```python
from build123d import *

# Parameters (mm, degrees)
CROQUIS1_W              = 43
CROQUIS1_H              = 15.5
SALIENTE_EXTRUIR1_DEPTH = 2
SALIENTE_EXTRUIR2_START = -2
SALIENTE_EXTRUIR2_DEPTH = 2


with BuildPart() as part:
    # Croquis1 → Saliente-Extruir1 (new body)
    with BuildSketch(Plane(origin=(0, 0, 0), x_dir=(1, 0, 0), z_dir=(0, 1, 0))):
        with BuildLine():
            Line((-24.5, 8.75), (-24.5, -8.75))
            ThreePointArc((-24.5, -8.75), (-23.914213562, -10.164213562), (-22.5, -10.75))
            Line((-22.5, -10.75), (22.5, -10.75))
            ThreePointArc((22.5, -10.75), (23.914213562, -10.164213562), (24.5, -8.75))
            Line((24.5, -8.75), (24.5, 8.75))
            ThreePointArc((24.5, 8.75), (23.914213562, 10.164213562), (22.5, 10.75))
            Line((22.5, 10.75), (-22.5, 10.75))
            ThreePointArc((-22.5, 10.75), (-23.914213562, 10.164213562), (-24.5, 8.75))
        make_face()
        Rectangle(CROQUIS1_W, CROQUIS1_H, mode=Mode.SUBTRACT)
    extrude(amount=SALIENTE_EXTRUIR1_DEPTH)

    # Croquis2 → Saliente-Extruir2 (add)
    with BuildSketch(Plane(origin=(0, 0, 0), x_dir=(1, 0, 0), z_dir=(0, 1, 0)).offset(SALIENTE_EXTRUIR2_START)):
        with BuildLine():
            Line((-24.5, 8.75), (-24.5, -8.75))
            ThreePointArc((-24.5, -8.75), (-23.914213562, -10.164213562), (-22.5, -10.75))
            Line((-22.5, -10.75), (22.5, -10.75))
            ThreePointArc((22.5, -10.75), (23.914213562, -10.164213562), (24.5, -8.75))
            Line((24.5, -8.75), (24.5, 8.75))
            ThreePointArc((24.5, 8.75), (23.914213562, 10.164213562), (22.5, 10.75))
            Line((22.5, 10.75), (-22.5, 10.75))
            ThreePointArc((-22.5, 10.75), (-23.914213562, 10.164213562), (-24.5, 8.75))
        make_face()
    extrude(amount=SALIENTE_EXTRUIR2_DEPTH)


solid = part.part
```
Design review of the part built by this model. Coordinates are the model's own, in mm. A direction names the side the tool comes from. Coordinates: 2 decimals unless noted, no trailing zeros. Loops run counter-clockwise (first coordinate to the right, second up) from the corner with the lowest first, then second, coordinate; pieces in that order, holes last.
Q1. We need section C-C on z = 4.25. State the section outline as (x, y) points, and give its area (3 significant figures).
Reported:
outline: (-24.5, -2) - (24.5, -2) - (24.5, 2) - (21.5, 2) - (21.5, 0) - (-21.5, 0) - (-21.5, 2) - (-24.5, 2) - close
area: 110 mm2
Q2. The part is to be moulded in two halves that separate along X. For faces 3 (the face through (-21.5, 1, 0)), 4 (the face through (-23.9, -0.03, -10.18)), 5 (the face through (0, 0, 10.75)), say which applies: +X half, -X half, draft (parallel to the pull), parting line (faces both ways), or undercut.
Reported:
face 3: undercut
face 4: -X half
face 5: draft
Q3. We need section A-A on y = 0.5. State the section outline as (x, z) points, and give its area (3 significant figures).
Reported:
outline: (-24.5, -8.75) arc R2 ccw to (-22.5, -10.75) - (22.5, -10.75) arc R2 ccw to (24.5, -8.75) - (24.5, 8.75) arc R2 ccw to (22.5, 10.75) - (-22.5, 10.75) arc R2 ccw to (-24.5, 8.75) - close; hole (-21.5, -7.75) - (21.5, -7.75) - (21.5, 7.75) - (-21.5, 7.75) - close
area: 384 mm2
Q4. Tool access review of faces 1 (the face through (0, 1, -7.75)), 2 (the face through (0, 0, -10.75)): name each direction out of +Z, -Z, +X, -X, +Y, -Y from which nothing blocks a thin tool from reaching the whole face with its end or side.
Reported:
face 1: +Y
face 2: -Z, +X, -X, +Y, -Y
Q5. We need section B-B on x = -14.5. State the section outline as (y, z) points, and give its area (3 significant figures).
Reported:
outline: (-2, -10.75) - (2, -10.75) - (2, -7.75) - (0, -7.75) - (0, 7.75) - (2, 7.75) - (2, 10.75) - (-2, 10.75) - close
area: 55.0 mm2
Q6. To check wall thickness, follow line 1 (Z direction, x = -14, y = 1.75); line 2 (X direction, y = 0.3, z = 0.5); line 3 (Y direction, x = -6.5, z = 1.75). State the ranges of each line that lie inside material, in increasing order.
Reported:
line 1: z = -10.75 to -7.75, 7.75 to 10.75
line 2: x = -24.5 to -21.5, 21.5 to 24.5
line 3: y = -2 to 0
